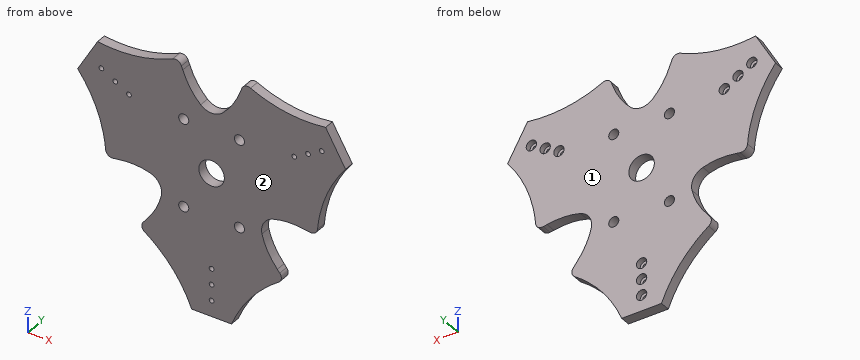
```python
from build123d import *

# Parameters (mm, degrees)
CROQUIS2_R            = 16
DELTA_BASE_DEPTH      = 12.7
CROQUIS3_R            = 3
CORTAR_EXTRUIR2_DEPTH = 30
CROQUIS5_R            = 6.5
CORTAR_EXTRUIR3_DEPTH = 7
CROQUIS6_R            = 6.35
CORTAR_EXTRUIR4_DEPTH = 38


with BuildPart() as part:
    # Croquis2 → Delta Base (new body)
    with BuildSketch(Plane(origin=(0, 0, 0), x_dir=(1, 0, 0), z_dir=(0, 1, 0))):
        with BuildLine():
            Line((168.384572854, -68.349364766), (143.384572854, -111.650634955))
            add(Edge.make_bspline(
                [(143.384572854, -111.650634955), (110.228964472, -106.994880788), (78.165264136, -111.818792753), (48.966207304, -125.543555732)],
                knots=[0, 0, 0, 0, 0.911575674, 0.911575674, 0.911575674, 0.911575674], degree=3))
            ThreePointArc((48.966207304, -125.543555732), (42.399289585, -125.651302831), (37.964762468, -120.806616359))
            add(Edge.make_bspline(
                [(36.219139152, -116.360829974), (36.873200125, -117.787733164), (37.457762294, -119.267608258), (37.964762468, -120.806616359)],
                knots=[0.875206919, 0.875206919, 0.875206919, 0.875206919, 0.919288331, 0.919288331, 0.919288331, 0.919288331], degree=3))
            add(Edge.make_bspline(
                [(36.219139152, -116.360829974), (31.103863708, -102.135589346), (23.600584995, -90.366962092), (13.709301605, -81.054947485)],
                knots=[0, 0, 0, 0, 0.49880396, 0.49880396, 0.49880396, 0.49880396], degree=3))
            ThreePointArc((13.709301605, -81.054947485), (4.34e-07, -75.617057833), (-13.709300808, -81.054947304))
            add(Edge.make_bspline(
                [(-36.219138946, -116.360830332), (-31.103863897, -102.135589743), (-23.600584693, -90.366962129), (-13.709300808, -81.054947304)],
                knots=[0, 0, 0, 0, 0.498803969, 0.498803969, 0.498803969, 0.498803969], degree=3))
            add(Edge.make_bspline(
                [(-36.219138946, -116.360830332), (-36.873199918, -117.787733522), (-37.457762087, -119.267608616), (-37.964762261, -120.806616717)],
                knots=[0.875206919, 0.875206919, 0.875206919, 0.875206919, 0.919288331, 0.919288331, 0.919288331, 0.919288331], degree=3))
            ThreePointArc((-37.964762261, -120.806616717), (-42.399289378, -125.651303189), (-48.966207097, -125.543556091))
            add(Edge.make_bspline(
                [(-143.384572647, -111.650635314), (-110.228964266, -106.994881146), (-78.165263929, -111.818793111), (-48.966207097, -125.543556091)],
                knots=[0, 0, 0, 0, 0.911575674, 0.911575674, 0.911575674, 0.911575674], degree=3))
            Line((-143.384572647, -111.650635314), (-168.384572647, -68.349365124))
            add(Edge.make_bspline(
                [(-168.384572647, -68.349365124), (-147.774767073, -41.963643072), (-135.920547212, -11.783708059), (-133.207012198, 20.365798414)],
                knots=[0, 0, 0, 0, 0.911575674, 0.911575674, 0.911575674, 0.911575674], degree=3))
            ThreePointArc((-133.207012198, 20.365798414), (-130.016865062, 26.106789533), (-123.603979946, 27.524859434))
            add(Edge.make_bspline(
                [(-118.881004339, 26.813720378), (-120.443769236, 26.960738555), (-122.017659747, 27.194430413), (-123.603979946, 27.524859434)],
                knots=[0.875206919, 0.875206919, 0.875206919, 0.875206919, 0.919288331, 0.919288331, 0.919288331, 0.919288331], degree=3))
            add(Edge.make_bspline(
                [(-118.881004339, 26.813720378), (-104.003947343, 24.131058268), (-90.060377482, 24.744774797), (-77.05029433, 28.654870325)],
                knots=[0, 0, 0, 0, 0.49880396, 0.49880396, 0.49880396, 0.49880396], degree=3))
            ThreePointArc((-77.05029433, 28.654870325), (-65.486293205, 37.808528635), (-63.340993077, 52.400076525))
            add(Edge.make_bspline(
                [(-82.6618656, 89.547109596), (-72.900083398, 78.004530603), (-66.459792532, 65.622186774), (-63.340993077, 52.400076525)],
                knots=[0, 0, 0, 0, 0.498803968, 0.498803968, 0.498803968, 0.498803968], degree=3))
            add(Edge.make_bspline(
                [(-82.6618656, 89.547109596), (-83.570569526, 90.826994609), (-84.559897867, 92.073177844), (-85.639217892, 93.281756925)],
                knots=[0.875206919, 0.875206919, 0.875206919, 0.875206919, 0.919288331, 0.919288331, 0.919288331, 0.919288331], degree=3))
            ThreePointArc((-85.639217892, 93.281756925), (-87.617575891, 99.544513298), (-84.240805308, 105.177757318))
            add(Edge.make_bspline(
                [(-25.000000207, 180.00000008), (-37.545803015, 148.95852386), (-57.75528349, 123.602500812), (-84.240805308, 105.177757318)],
                knots=[0, 0, 0, 0, 0.911575674, 0.911575674, 0.911575674, 0.911575674], degree=3))
            Line((-25.000000207, 180.00000008), (24.999999793, 180.00000008))
            add(Edge.make_bspline(
                [(24.999999793, 180.00000008), (37.545802601, 148.95852386), (57.755283076, 123.602500812), (84.240804894, 105.177757318)],
                knots=[0, 0, 0, 0, 0.911575674, 0.911575674, 0.911575674, 0.911575674], degree=3))
            ThreePointArc((84.240804894, 105.177757318), (87.617575478, 99.544513298), (85.639217478, 93.281756925))
            add(Edge.make_bspline(
                [(82.661865187, 89.547109596), (83.570569112, 90.826994609), (84.559897453, 92.073177844), (85.639217478, 93.281756925)],
                knots=[0.875206919, 0.875206919, 0.875206919, 0.875206919, 0.919288331, 0.919288331, 0.919288331, 0.919288331], degree=3))
            add(Edge.make_bspline(
                [(82.661865187, 89.547109596), (72.90008315, 78.0045308), (66.459792337, 65.622187196), (63.340992822, 52.400077201)],
                knots=[0, 0, 0, 0, 0.49880396, 0.49880396, 0.49880396, 0.49880396], degree=3))
            ThreePointArc((63.340992822, 52.400077201), (65.486292826, 37.808529293), (77.050293872, 28.654870884))
            add(Edge.make_bspline(
                [(118.881004546, 26.813720736), (104.003947297, 24.131058581), (90.060377214, 24.744775176), (77.050293872, 28.654870884)],
                knots=[0, 0, 0, 0, 0.498803969, 0.498803969, 0.498803969, 0.498803969], degree=3))
            add(Edge.make_bspline(
                [(118.881004546, 26.813720736), (120.443769443, 26.960738913), (122.017659954, 27.194430772), (123.603980153, 27.524859792)],
                knots=[0.875206919, 0.875206919, 0.875206919, 0.875206919, 0.919288331, 0.919288331, 0.919288331, 0.919288331], degree=3))
            ThreePointArc((123.603980153, 27.524859792), (130.016865269, 26.106789891), (133.207012404, 20.365798772))
            add(Edge.make_bspline(
                [(168.384572854, -68.349364766), (147.77476728, -41.963642714), (135.920547419, -11.783707701), (133.207012404, 20.365798772)],
                knots=[0, 0, 0, 0, 0.911575674, 0.911575674, 0.911575674, 0.911575674], degree=3))
        make_face()
        with Locations(Location((-2.07e-07, 8e-08, 0), (0, 0, 270))):
            Circle(CROQUIS2_R, mode=Mode.SUBTRACT)
    extrude(amount=DELTA_BASE_DEPTH)

    # Croquis3 → Cortar-Extruir2 (cut)
    with BuildSketch(Plane(origin=(0, 12.7, 0), x_dir=(1, 0, 0), z_dir=(0, 1, 0))):
        with Locations(Location((0, 120, 0), (0, 0, 270))):
            Circle(CROQUIS3_R)
        with Locations(Location((0, 140, 0), (0, 0, 270))):
            Circle(CROQUIS3_R)
        with Locations(Location((0, 160, 0), (0, 0, 270))):
            Circle(CROQUIS3_R)
        with Locations(Location((103.923048454, -60, 0), (0, 0, 270))):
            Circle(CROQUIS3_R)
        with Locations(Location((121.24355653, -70, 0), (0, 0, 270))):
            Circle(CROQUIS3_R)
        with Locations(Location((138.564064606, -80, 0), (0, 0, 270))):
            Circle(CROQUIS3_R)
        with Locations(Location((-103.923048454, -60, 0), (0, 0, 270))):
            Circle(CROQUIS3_R)
        with Locations(Location((-121.24355653, -70, 0), (0, 0, 270))):
            Circle(CROQUIS3_R)
        with Locations(Location((-138.564064605, -80, 0), (0, 0, 270))):
            Circle(CROQUIS3_R)
    extrude(amount=-CORTAR_EXTRUIR2_DEPTH, mode=Mode.SUBTRACT)

    # Croquis5 → Cortar-Extruir3 (cut)
    with BuildSketch(Plane(origin=(0, 12.7, 0), x_dir=(1, 0, 0), z_dir=(0, 1, 0))):
        with Locations(Location((0, 160, 0), (0, 0, 270))):
            Circle(CROQUIS5_R)
        with Locations(Location((0, 140, 0), (0, 0, 270))):
            Circle(CROQUIS5_R)
        with Locations(Location((0, 120, 0), (0, 0, 270))):
            Circle(CROQUIS5_R)
        with Locations(Location((138.564064606, -80, 0), (0, 0, 270))):
            Circle(CROQUIS5_R)
        with Locations(Location((121.24355653, -70, 0), (0, 0, 270))):
            Circle(CROQUIS5_R)
        with Locations(Location((103.923048454, -60, 0), (0, 0, 270))):
            Circle(CROQUIS5_R)
        with Locations(Location((-138.564064606, -80, 0), (0, 0, 270))):
            Circle(CROQUIS5_R)
        with Locations(Location((-121.24355653, -70, 0), (0, 0, 270))):
            Circle(CROQUIS5_R)
        with Locations(Location((-103.923048454, -60, 0), (0, 0, 270))):
            Circle(CROQUIS5_R)
    extrude(amount=-CORTAR_EXTRUIR3_DEPTH, mode=Mode.SUBTRACT)

    # Croquis6 → Cortar-Extruir4 (cut)
    with BuildSketch(Plane(origin=(0, 12.7, 0), x_dir=(1, 0, 0), z_dir=(0, 1, 0))):
        with Locations(Location((-35, 55, 0), (0, 0, 270))):
            Circle(CROQUIS6_R)
        with Locations(Location((35, 55.00000008, 0), (0, 0, 270))):
            Circle(CROQUIS6_R)
        with Locations(Location((-35, -55, 0), (0, 0, 270))):
            Circle(CROQUIS6_R)
        with Locations(Location((35, -55, 0), (0, 0, 270))):
            Circle(CROQUIS6_R)
    extrude(amount=-CORTAR_EXTRUIR4_DEPTH, mode=Mode.SUBTRACT)


solid = part.part
```
The model under review builds one solid part; all positions refer to its coordinate system, in mm. Face numbers are marked on the shaded views. Round coordinates to 2 decimals unless told otherwise and drop trailing zeros. Use CSV: the item, a comma, the result in double quotes. Start each with the question number.
(1) We need section A-A, the plane y = 8. State how many separate pieces and enclosed holes the cut face has, then the cut area to 3 significant figures.
(2) For line 1 along X through (y, z) = (7, 55); line 2 along X through (y, z) = (1.45, 80); line 3 along X through (y, z) = (9.5, 80), list the stretches that pass through material, from the lowest coordinate up.
(3) Clearance check with flat-ended pins moving along their axes: P1, Ø4, axis at x = -105, z = 60, coming from the +Y side; P2, Ø6, axis at x = 79, y = 2, coming from the -Z side; P3, Ø1, axis at y = 4, z = -55.5, coming from the +X side; P4, Ø11.5, axis at x = 35, z = -55, coming from the -Y side. State where each tip first meets the part, or that it passes through.
(4) The part is to be moulded in two halves that separate along Y. For the marked faces 1 and 2, say which applies: +Y half, -Y half, draft (parallel to the pull), parting line (faces both ways), or undercut.
Findings:
1,separate pieces,"1"
1,enclosed holes,"14"
1,area,"56,200 mm^2"
2,line 1,"-158.91 to -108.08, -99.77 to -41.35, -28.65 to 28.65, 41.35 to 99.77, 108.08 to 158.91"
2,line 2,"-161.66 to -141.56, -135.56 to -12.49, 12.49 to 135.56, 141.56 to 161.66"
2,line 3,"-161.66 to -145.06, -132.06 to -12.49, 12.49 to 132.06, 145.06 to 161.66"
3,P1,"y = 5.7"
3,P2,"z = -111.29"
3,P3,"x = 64.28"
3,P4,"through"
4,face 1,"+Y half"
4,face 2,"-Y half"
